Verification items for the finished model (mm, model axes). Face numbers are marked on the shaded views. A direction names the side the tool comes from. Round coordinates to 2 decimals unless told otherwise and drop trailing zeros. Write each loop counter-clockwise with the first axis right and the second up, starting at its lowest first coordinate (ties: lowest second). Pieces come first, ordered by that corner, then holes. Notation, with made-up numbers: (-27.75, -20) - (27.25, -20) arc R29 cw to (27.25, 18) - close; hole circle Ø11 at (12.5, 18.25). An arc over 180 degrees is marked (long way). Answer as a JSON object with one key per item and string values.
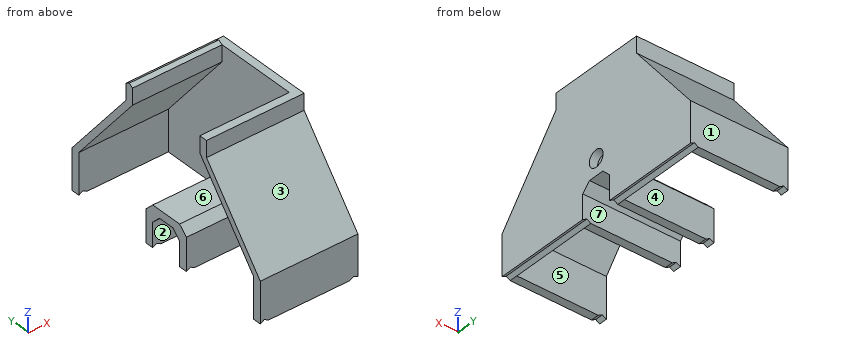
```python
from build123d import *

# Parameters (mm, degrees)
EXTRUDE014_DEPTH = 100
EXTRUDE010_DEPTH = 22
SKETCH009_R      = 4.125
EXTRUDE011_DEPTH = 4


with BuildPart() as extrude014:
    # Sketch012 → Extrude014 (new body, symmetric)
    with BuildSketch(Plane.XZ):
        Polygon((-20, 0), (-24, 0), (-22, 1.154701), align=None)
        Polygon((20, 0), (22, 1.154701), (24, 0), align=None)
    extrude(amount=EXTRUDE014_DEPTH, both=True)


with BuildPart() as extrude014_1:
    # Extrude014 placement: moved
    add(extrude014.part.moved(Location((1, 0, -20))))


with BuildPart() as extrude010:
    # Sketch008 → Extrude010 (new body, symmetric)
    with BuildSketch(Plane.YZ):
        Polygon((-56, 0), (-24, 40), (-24, 48), (-20, 48), (-20, 40), (-52, 0), (-52, -20), (-56, -20), align=None)
        Polygon((52, 0), (20, 40), (20, 48), (22, 49.154701), (24, 48), (24, 40), (56, 0), (56, -20), (52, -20), align=None)
        Polygon((-8, -20), (-12, -20), (-12, -4), (-8, 0), (8, 0), (12, -4), (12, -20), (8, -20), (8, -8), (4, -4), (-4, -4), (-8, -8), align=None)
    extrude(amount=EXTRUDE010_DEPTH, both=True)


with BuildPart() as stage_1_paths:
    # Sketch009 → Extrude011 (new body)
    with BuildSketch(Plane.YZ):
        Polygon((-56, 0), (-24, 40), (-24, 48), (24, 48), (24, 40), (56, 0), (56, -20), (52, -20), (12, -20), (8, -20), (8, -8), (4, -4), (-4, -4), (-8, -8), (-8, -20), (-12, -20), (-52, -20), (-56, -20), align=None)
        with Locations((0, 4.125)):
            Circle(SKETCH009_R, mode=Mode.SUBTRACT)
    extrude(amount=EXTRUDE011_DEPTH)


with BuildPart() as stage_1_paths_1:
    # Extrude011 placement: moved
    add(stage_1_paths.part.moved(Location((22, 0, 0))))

    # Fusion006: union Extrude010
    add(extrude010.part)


with BuildPart() as stage_1_paths_2:
    # Fusion006 placement: moved
    add(stage_1_paths_1.part.moved(Location((-1, 0, 0))))

    # Cut: cut Extrude014
    add(extrude014_1.part, mode=Mode.SUBTRACT)


solid = stage_1_paths_2.part
```
Q1. Section check A-A, the plane z = -12. Record the cut outline in (x, y), then the cut area to 3 significant figures.
Geometry check:
{"outline": "(-23, -56) - (25, -56) - (25, -8) - (-23, -8) - (-23, -12) - (21, -12) - (21, -52) - (-23, -52) - close; (-23, 8) - (25, 8) - (25, 56) - (-23, 56) - (-23, 52) - (21, 52) - (21, 12) - (-23, 12) - close", "area": "1,090 mm2"}
Q2. Material ranges on line 1 along Z through (x, y) = (22.6, 0); line 2 along Y through (x, z) = (5, -1); line 3 along Y through (x, z) = (8, -13.5), recorded low to high. Write a range as [from, to].
Geometry check:
{"line 1": "z = [-4, 0], [8.25, 48]", "line 2": "y = [-56, -52], [-9, 9], [52, 56]", "line 3": "y = [-56, -52], [-12, -8], [8, 12], [52, 56]"}
Q3. Section check B-B, the plane x = 11.5. State how many separate pieces and enclosed holes the cut face has, then the cut area to 3 significant figures.
Geometry check:
{"separate pieces": "3", "enclosed holes": "0", "area": "770 mm2"}
Q4. Release check for a two-part mould opening along Y. For the marked faces 1, 2 and 3 record: released by +Y, released by -Y, zero draft, split by the parting line, or undercut.
Geometry check:
{"face 1": "released by +Y", "face 2": "undercut", "face 3": "released by -Y"}
Q5. Set-up check for the marked faces 4, 5, 6 and 7: record each of +Z, -Z, +X, -X, +Y, -Y from which the full face is reachable in a straight line by a thin tool's end or side.
Geometry check:
{"face 4": "+Z, -Z, -X", "face 5": "-Z, -X", "face 6": "+Z, -X", "face 7": "-Z, +X, -X"}
Q6. Gauge pin test, flat ends, axial feed: P1, Ø10, axis at x = -5.5, y = 17.5, coming from the -Z side (3 decimals); P2, Ø6.5, axis at x = 10.5, z = 44.5, coming from the +Y side; P3, Ø1.5, axis at y = 14, z = 42, coming from the -X side. Record the tip position at first contact, or that the pin passes through.
Geometry check:
{"P1": "stops at z = 36.875", "P2": "stops at y = 24", "P3": "stops at x = 21"}
Q7. Section check D-D, the plane z = 35.5. Record the cut outline in (x, y).
Geometry check:
{"outline": "(-23, -27.6) - (25, -27.6) - (25, 27.6) - (-23, 27.6) - (-23, 23.6) - (21, 23.6) - (21, -23.6) - (-23, -23.6) - close"}
Q8. Section check C-C, the plane y = -47. Record the cut outline in (x, z).
Geometry check:
{"outline": "(-23, 6.25) - (21, 6.25) - (21, -20) - (23, -18.85) - (25, -20) - (25, 11.25) - (-23, 11.25) - close"}
